Drawing for the job (mm, zero at the part's lowest x, y, z). A direction names the side the tool comes from. Give positions to 0.01 mm unless a question says otherwise; leave off trailing zeros. Write each loop counter-clockwise with the first axis right and the second up, starting at its lowest first coordinate (ties: lowest second). Pieces come first, ordered by that corner, then holes. Notation, with made-up numbers: M 74.25,16.5 L 112.25,16.5 A9 ccw 112.25,32.5 Z; hole C -7,-13 d3. An arc over 180 degrees is marked long. Use CSV: the item, a comma, the result in double quotes. Start each with the question number.
1. Band-saw the part on D-D, the plane z = 69.5. List the corners of the cut face in (x, y).
2. Drop flat-ended pins along their axis: pin 1 Ø5 at (y, z) = (39.5, 21.5) entering from -X; pin 2 Ø5 at (x, z) = (43, 68) entering from +Y; pin 3 Ø8 at (y, z) = (7.5, 46.5) entering from +X; pin 4 Ø16 at (x, y) = (35.5, 44.5) entering from -Z. Give the stop position or say it passes through.
3. Band-saw the part on C-C, the plane x = 34. List the corners of the cut face in (y, z), then the cut area to 3 significant figures.
4. Drill centre line: line 1 along X through (y, z) = (32, 72). Where is it in solid material? Low to high. Write a range as from..to.
5. 3-axis set-ups, long thin cutter, end or side, ignore diameter. For the marked faces 1, 2, 3, 4 and 5: which of +Z, -Z, +X, -X, +Y, -Y reach the whole face in a straight line?
6. Band-saw the part on A-A, the plane z = 47. List the corners of the cut face in (x, y), then the cut area to 3 significant figures.
7. Band-saw the part on B-B, the plane y = 33.5. List the corners of the cut face in (x, z).
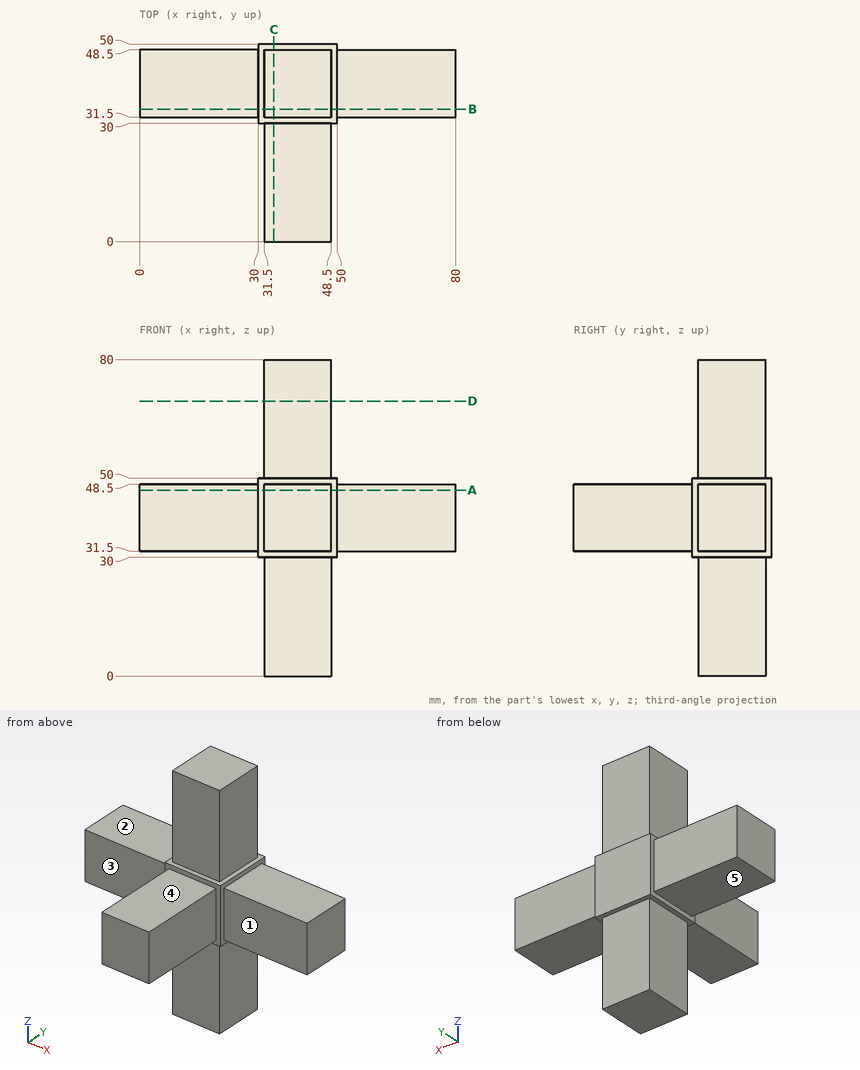
Output:
1,outline,"M 31.5,31.5 L 48.5,31.5 L 48.5,48.5 L 31.5,48.5 Z"
2,pin 1,"stops at x = 31.5"
2,pin 2,"stops at y = 48.5"
2,pin 3,"stops at x = 48.5"
2,pin 4,"stops at z = 0"
3,outline,"M 0,31.5 L 30,31.5 L 30,30 L 31.5,30 L 31.5,0 L 48.5,0 L 48.5,30 L 50,30 L 50,50 L 48.5,50 L 48.5,80 L 31.5,80 L 31.5,50 L 30,50 L 30,48.5 L 0,48.5 Z"
3,area,"1,930 mm²"
4,line 1,"x = 31.5..48.5"
5,face 1,"+Z, -Z, +X, -Y"
5,face 2,"+Z, -X, +Y, -Y"
5,face 3,"+Z, -Z, -X, -Y"
5,face 4,"+Z, +X, -X, -Y"
5,face 5,"-Z, -X, +Y, -Y"
6,outline,"M 0,31.5 L 30,31.5 L 30,30 L 31.5,30 L 31.5,0 L 48.5,0 L 48.5,30 L 50,30 L 50,31.5 L 80,31.5 L 80,48.5 L 50,48.5 L 50,50 L 30,50 L 30,48.5 L 0,48.5 Z"
6,area,"1,930 mm²"
7,outline,"M 0,31.5 L 30,31.5 L 30,30 L 31.5,30 L 31.5,0 L 48.5,0 L 48.5,30 L 50,30 L 50,31.5 L 80,31.5 L 80,48.5 L 50,48.5 L 50,50 L 48.5,50 L 48.5,80 L 31.5,80 L 31.5,50 L 30,50 L 30,48.5 L 0,48.5 Z"
